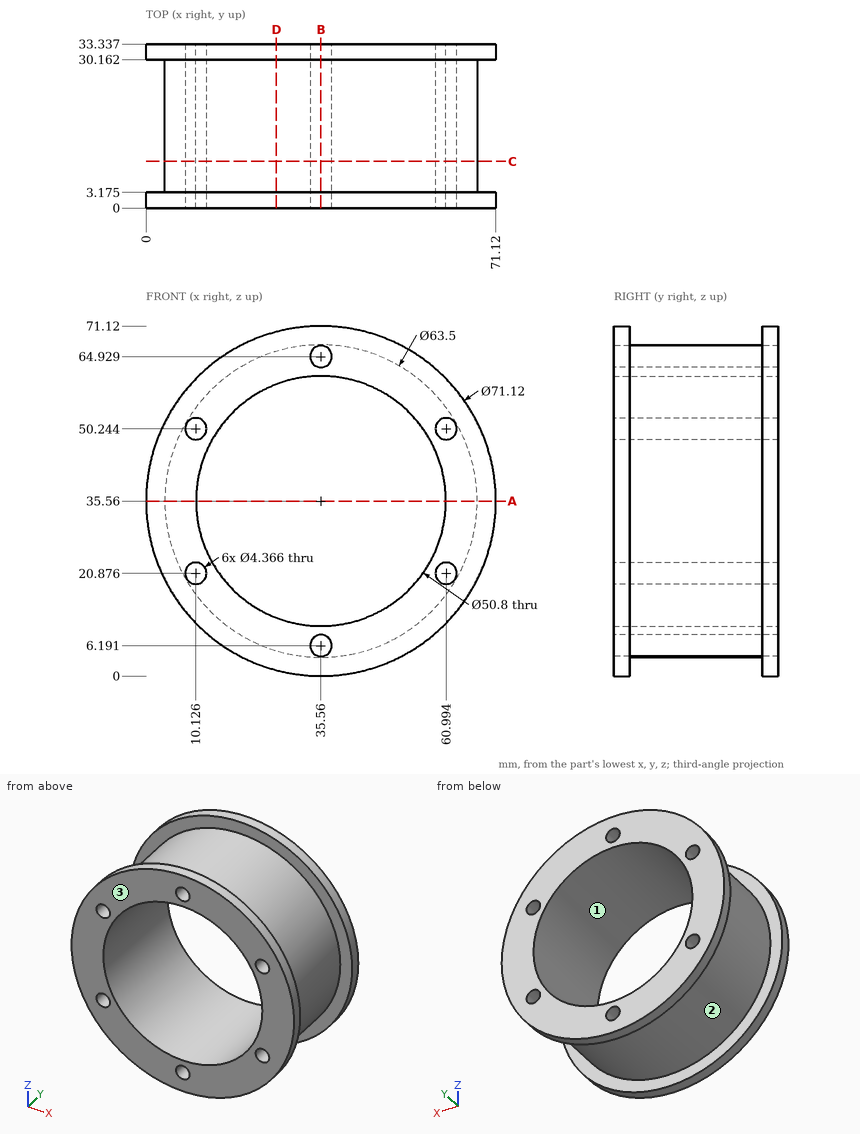
Source: three-view drawing plus pictorial views. Frame: mm from the lowest corner of the part. Give positions to 0.01 mm unless a question says otherwise; leave off trailing zeros. Write each loop counter-clockwise with the first axis right and the second up, starting at its lowest first coordinate (ties: lowest second). Pieces come first, ordered by that corner, then holes.
(1) Cut plane B-B, the plane x = 35.56. Return loops of the section in (y, z) (1 decimal).
(2) Mould query, pull axis Z, two halves, no side actions, for the marked faces 1, 2 and 3. Classes: released by +Z, released by -Z, zero draft, split by the parting line, or undercut.
(3) Cut plane D-D, the plane x = 26.5. Return loops of the section in (y, z) (1 decimal).
(4) Ray query, line 1 (Z direction, x = 35.56, y = 22.5) (1 decimal); line 2 (Z direction, x = 34.5, y = 27); line 3 (Y direction, x = 52.5, z = 65.5) (1 decimal). Return the intervals inside material, ascending.
(5) Cut plane A-A, the plane z = 35.56. Return loops of the section in (x, y) (1 decimal).
(6) First-contact query: P1, Ø6, axis at y = 21.5, z = 45.5, coming from the +X side; P2, Ø5, axis at x = 39, y = 19, coming from the +Z side; P3, Ø3.5, axis at x = 60.99, z = 20.88, coming from the +Y side; P4, Ø8, axis at y = 5.5, z = 38.5, coming from the -X side. Flat tips, straight axial feed; report the tip coordinate or a pass-through.
(7) Cut plane C-C, the plane y = 9.5. Give the number of separate pieces and of enclosed holes in the cut face, then the cut area to 3 significant figures.
Values follow:
1. outline: (0, 0) - (3.2, 0) - (3.2, 3.8) - (30.2, 3.8) - (30.2, 0) - (33.3, 0) - (33.3, 4) - (0, 4) - close; (0, 8.4) - (33.3, 8.4) - (33.3, 10.2) - (0, 10.2) - close; (0, 61) - (33.3, 61) - (33.3, 62.7) - (0, 62.7) - close; (0, 67.1) - (33.3, 67.1) - (33.3, 71.1) - (30.2, 71.1) - (30.2, 67.3) - (3.2, 67.3) - (3.2, 71.1) - (0, 71.1) - close
2. face 1: undercut
2. face 2: split by the parting line
2. face 3: zero draft
3. outline: (0, 1.2) - (3.2, 1.2) - (3.2, 5.1) - (30.2, 5.1) - (30.2, 1.2) - (33.3, 1.2) - (33.3, 11.8) - (0, 11.8) - close; (0, 59.3) - (33.3, 59.3) - (33.3, 69.9) - (30.2, 69.9) - (30.2, 66) - (3.2, 66) - (3.2, 69.9) - (0, 69.9) - close
4. line 1: z = 3.8 to 4, 8.4 to 10.2, 61 to 62.7, 67.1 to 67.3
4. line 2: z = 3.83 to 4.28, 8.1 to 10.18, 60.94 to 63.02, 66.84 to 67.29
4. line 3: y = 0 to 3.2, 30.2 to 33.3
5. outline: (0, 0) - (10.2, 0) - (10.2, 33.3) - (0, 33.3) - (0, 30.2) - (3.8, 30.2) - (3.8, 3.2) - (0, 3.2) - close; (61, 0) - (71.1, 0) - (71.1, 3.2) - (67.3, 3.2) - (67.3, 30.2) - (71.1, 30.2) - (71.1, 33.3) - (61, 33.3) - close
6. P1: stops at x = 66.54
6. P2: stops at z = 67.3
6. P3: passes through
6. P4: stops at x = 0
7. separate pieces: 1
7. enclosed holes: 7
7. area: 1,050 mm2
